Here's the drawing with two shaded views (mm, measured from the low corner). I have some questions. A direction names the side the tool comes from. Round coordinates to 2 decimals unless told otherwise and drop trailing zeros. Order: outer loops, then holes, each group sorted by start corner. A loop starts at its lowest first (then second) coordinate and runs counter-clockwise, first axis right, second up. Notation, with made-up numbers: (62, -26.75) -> (75, -26.75) arc R19 ccw to (75, 8.25) -> close; hole circle Ø4 at (5.5, 29). An arc over 180 degrees is marked (long way). One line per question, with ' | ' between items.
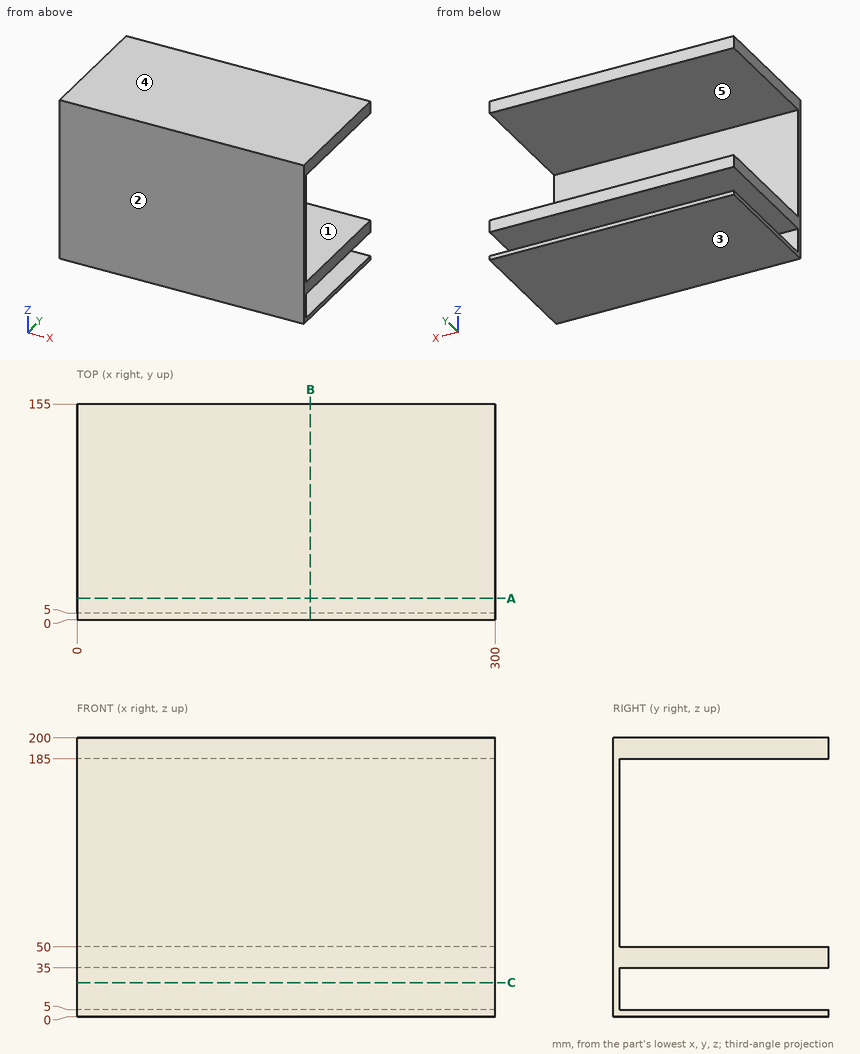
1. I need wall thicknesses on probe 1 along Z at (x, y) = (117, 103); probe 2 along Y at (x, z) = (194, 172.5). Which ranges of each line are inside material? Lowest first, please.
From the geometry:
probe 1: z = 0 to 5, 35 to 50, 185 to 200 | probe 2: y = 0 to 5
2. I want a section at C-C on z = 24.5. List the corners of the cut face in (x, y) for me.
From the geometry:
outline: (0, 0) -> (300, 0) -> (300, 5) -> (0, 5) -> close
3. I want a section at B-B on x = 167.5. List the corners of the cut face in (y, z) for me, and give its area (3 significant figures).
From the geometry:
outline: (0, 0) -> (155, 0) -> (155, 5) -> (5, 5) -> (5, 35) -> (155, 35) -> (155, 50) -> (5, 50) -> (5, 185) -> (155, 185) -> (155, 200) -> (0, 200) -> close | area: 6,250 mm²
4. If we mould it in two halves opening along Z, with no side actions, what happens to the marked faces 1, 2 and 3? For each: pulls with the +Z half, pulls with the -Z half, needs draft (parallel to the pull), parting line crosses it, or undercut.
From the geometry:
face 1: undercut | face 2: needs draft | face 3: pulls with the -Z half
5. I want a section at A-A on y = 15.5. List the corners of the cut face in (x, z) for me, and give its area (3 significant figures).
From the geometry:
outline: (0, 0) -> (300, 0) -> (300, 5) -> (0, 5) -> close; (0, 35) -> (300, 35) -> (300, 50) -> (0, 50) -> close; (0, 185) -> (300, 185) -> (300, 200) -> (0, 200) -> close | area: 10,500 mm²
6. On a 3-axis mill with a long thin cutter (end or side, diameter ignored), from which of +Z, -Z, +X, -X, +Y, -Y can I reach the whole of each face in a straight line? I mean the marked faces 4 and 5. Say none if no direction works.
From the geometry:
face 4: +Z, +X, -X, +Y, -Y | face 5: +X, -X, +Y
7. I'm going to push flat-ended pins straight in: pin 1 (1 mm diameter, centred on x = 260.5, z = 117.5, fed in from -Y); pin 2 (9 mm diameter, centred on x = 161, z = 24.5, fed in from +Y). Where does each tip first touch, or does it pass through?
From the geometry:
pin 1: stops at y = 0 | pin 2: stops at y = 5
